```python
from build123d import *

# Parameters (mm, degrees)
SKETCH1_R           = 40
SKETCH1_R_2         = 2.575
BOSS_EXTRUDE1_DEPTH = 7.5


with BuildPart() as part:
    # Sketch1 → Boss-Extrude1 (new body)
    with BuildSketch(Plane(origin=(0, 0, 0), x_dir=(1, 0, 0), z_dir=(0, 1, 0))):
        with Locations(Location((0, 0, 0), (0, 0, 270))):
            Circle(SKETCH1_R)
        with Locations(Location((0, 0, 0), (0, 0, 270))):
            Circle(SKETCH1_R_2, mode=Mode.SUBTRACT)
        with BuildLine():
            Line((-2.575, 11.423413457), (-2.575, 29.027906831))
            ThreePointArc((-2.575, 29.027906831), (-4.518245185, 32.984704779), (-8.8375, 33.865891303))
            ThreePointArc((-8.8375, 33.865891303), (-20.57248383, 28.315594803), (-29.477438916, 18.870097905))
            ThreePointArc((-29.477438916, 18.870097905), (-29.974103871, 14.489940856), (-26.811461186, 11.419087051))
            Line((-26.811461186, 11.419087051), (-10.068593046, 5.978999421))
            ThreePointArc((-10.068593046, 5.978999421), (-8.648029574, 5.942087171), (-7.436840448, 6.68531257))
            ThreePointArc((-7.436840448, 6.68531257), (-5.877852523, 8.090169944), (-4.06, 9.138730765))
            ThreePointArc((-4.06, 9.138730765), (-2.978872618, 10.060970797), (-2.575, 11.423413457))
        make_face(mode=Mode.SUBTRACT)
        with BuildLine():
            Line((2.575, 11.423413457), (2.575, 29.027906831))
            ThreePointArc((2.575, 29.027906831), (4.518245185, 32.984704779), (8.8375, 33.865891303))
            ThreePointArc((8.8375, 33.865891303), (20.57248383, 28.315594803), (29.477438916, 18.870097905))
            ThreePointArc((29.477438916, 18.870097905), (29.974103871, 14.489940856), (26.811461186, 11.419087051))
            Line((26.811461186, 11.419087051), (10.068593046, 5.978999421))
            ThreePointArc((10.068593046, 5.978999421), (8.648029574, 5.942087171), (7.436840448, 6.68531257))
            ThreePointArc((7.436840448, 6.68531257), (5.877852523, 8.090169944), (4.06, 9.138730765))
            ThreePointArc((4.06, 9.138730765), (2.978872618, 10.060970797), (2.575, 11.423413457))
        make_face(mode=Mode.SUBTRACT)
        with BuildLine():
            Line((11.660030567, 1.081058362), (28.402898707, 6.521145993))
            ThreePointArc((28.402898707, 6.521145993), (32.766532965, 5.895727806), (34.939314292, 2.06017398))
            ThreePointArc((34.939314292, 2.06017398), (33.28697807, -10.815594803), (27.055559151, -22.203529427))
            ThreePointArc((27.055559151, -22.203529427), (23.04326016, -24.029428835), (19.145394301, -21.970522913))
            Line((19.145394301, -21.970522913), (8.797732721, -7.728188595))
            ThreePointArc((8.797732721, -7.728188595), (8.323648831, -6.388558961), (8.656220166, -5.006980372))
            ThreePointArc((8.656220166, -5.006980372), (9.510565163, -3.090169944), (9.946058442, -1.037266343))
            ThreePointArc((9.946058442, -1.037266343), (10.4890741, 0.275934741), (11.660030567, 1.081058362))
        make_face(mode=Mode.SUBTRACT)
        with BuildLine():
            Line((4.6312952, -10.755282645), (14.97895678, -24.997616962))
            ThreePointArc((14.97895678, -24.997616962), (15.732585881, -29.340944607), (12.756183776, -32.592633761))
            ThreePointArc((12.756183776, -32.592633761), (0, -35), (-12.756183776, -32.592633761))
            ThreePointArc((-12.756183776, -32.592633761), (-15.732585881, -29.340944607), (-14.97895678, -24.997616962))
            Line((-14.97895678, -24.997616962), (-4.6312952, -10.755282645))
            ThreePointArc((-4.6312952, -10.755282645), (-3.503731686, -9.890433748), (-2.087002171, -9.77979662))
            ThreePointArc((-2.087002171, -9.77979662), (0, -10), (2.087002171, -9.77979662))
            ThreePointArc((2.087002171, -9.77979662), (3.503731686, -9.890433748), (4.6312952, -10.755282645))
        make_face(mode=Mode.SUBTRACT)
        with BuildLine():
            Line((-8.797732721, -7.728188595), (-19.145394301, -21.970522913))
            ThreePointArc((-19.145394301, -21.970522913), (-23.04326016, -24.029428835), (-27.055559151, -22.203529427))
            ThreePointArc((-27.055559151, -22.203529427), (-33.28697807, -10.815594803), (-34.939314292, 2.06017398))
            ThreePointArc((-34.939314292, 2.06017398), (-32.766532965, 5.895727806), (-28.402898707, 6.521145993))
            Line((-28.402898707, 6.521145993), (-11.660030567, 1.081058362))
            ThreePointArc((-11.660030567, 1.081058362), (-10.4890741, 0.275934741), (-9.946058442, -1.037266343))
            ThreePointArc((-9.946058442, -1.037266343), (-9.510565163, -3.090169944), (-8.656220166, -5.006980372))
            ThreePointArc((-8.656220166, -5.006980372), (-8.323648831, -6.388558961), (-8.797732721, -7.728188595))
        make_face(mode=Mode.SUBTRACT)
    extrude(amount=BOSS_EXTRUDE1_DEPTH)


solid = part.part
```
Work out the finished part from the listing and answer in its coordinate system (mm). Round coordinates to 2 decimals unless told otherwise and drop trailing zeros. Order: outer loops, then holes, each group sorted by start corner. A loop starts at its lowest first (then second) coordinate and runs counter-clockwise, first axis right, second up.
Q1. A cutting plane is placed at A-A, the plane x = 0. Determine the outline of the cut face in (y, z) (3 decimals), then the cut area to 3 significant figures.
Solution:
outline: (0, -40) - (7.5, -40) - (7.5, -2.575) - (0, -2.575) - close; (0, 2.575) - (7.5, 2.575) - (7.5, 10) - (0, 10) - close; (0, 35) - (7.5, 35) - (7.5, 40) - (0, 40) - close
area: 374 mm2
Q2. Given pin 1 Ø2 at (y, z) = (3, -16) entering from -X; pin 2 Ø2 at (y, z) = (2, -23) entering from +X; pin 3 Ø8 at (x, z) = (0, 0) entering from -Y; pin 4 Ø3 at (y, z) = (2, 30.5) entering from -X, each flat-ended and moving along its own axis, determine where each tip first touches the part or whether it passes through.
Solution:
pin 1: stops at x = -37.08
pin 2: stops at x = 33.41
pin 3: stops at y = 0
pin 4: stops at x = -27.55
Q3. A cutting plane is placed at B-B, the plane z = -4. Determine the outline of the cut face in (x, y), then the cut area to 3 significant figures.
Solution:
outline: (-39.8, 0) - (-34.42, 0) - (-34.42, 7.5) - (-39.8, 7.5) - close; (-20.64, 0) - (20.64, 0) - (20.64, 7.5) - (-20.64, 7.5) - close; (34.42, 0) - (39.8, 0) - (39.8, 7.5) - (34.42, 7.5) - close
area: 390 mm2
Q4. Find the intervals of material crossed by line 1 along X through (y, z) = (4, 0) (3 decimals); line 2 along Z through (x, y) = (-6, 2); line 3 along X through (y, z) = (5.5, -20) (3 decimals), in increasing order.
Solution:
line 1: x = -40 to -35, -10.295 to -2.575, 2.575 to 10.295, 35 to 40
line 2: z = -39.55 to -33.77, -8 to 12.64, 34.48 to 39.55
line 3: x = -34.641 to -28.723, -2.575 to 2.575, 28.723 to 34.641
Q5. A cutting plane is placed at C-C, the plane x = -32. Determine the outline of the cut face in (y, z).
Solution:
outline: (0, -24) - (7.5, -24) - (7.5, -6.33) - (0, -6.33) - close; (0, 14.18) - (7.5, 14.18) - (7.5, 24) - (0, 24) - close
Q6. A cutting plane is placed at D-D, the plane y = 3.75. Count the separate pieces of the cut face and the enclosed holes in it, then the cut area to 3 significant figures.
Solution:
separate pieces: 1
enclosed holes: 6
area: 2,210 mm2
